from build123d import *

# Parameters (mm, degrees)
F0_W     = 19.05
F0_H     = 152.4
F0_W_2   = 304.8
F0_H_2   = 38.1
F1_DEPTH = 19.05


with BuildPart() as f1:
    # F0 (on Front) → F1 (new body)
    with BuildSketch(Plane.XZ):
        Polygon((-438.15, -314.325), (-438.15, -447.675), (-152.4, -447.675), (152.4, -447.675), (438.15, -447.675), (438.15, -314.325), (438.15, -161.925), (438.15, 142.875), (438.15, 295.275), (438.15, 447.675), (357.716667, 447.675), (357.716667, 422.275), (338.666667, 422.275), (338.666667, 447.675), (258.233333, 447.675), (258.233333, 422.275), (239.183333, 422.275), (239.183333, 447.675), (158.75, 447.675), (158.75, 422.275), (139.7, 422.275), (139.7, 447.675), (59.266667, 447.675), (59.266667, 422.275), (40.216667, 422.275), (40.216667, 447.675), (-40.216667, 447.675), (-40.216667, 422.275), (-59.266667, 422.275), (-59.266667, 447.675), (-139.7, 447.675), (-139.7, 422.275), (-158.75, 422.275), (-158.75, 447.675), (-239.183333, 447.675), (-239.183333, 422.275), (-258.233333, 422.275), (-258.233333, 447.675), (-338.666667, 447.675), (-338.666667, 422.275), (-357.716667, 422.275), (-357.716667, 447.675), (-438.15, 447.675), (-438.15, 295.275), (-438.15, 142.875), (-438.15, -161.925), align=None)
        Polygon((-304.00625, -193.675), (-304.00625, -117.475), (305.59375, -117.475), (305.59375, -193.675), (305.59375, -231.775), (286.54375, -231.775), (286.54375, -193.675), (207.16875, -193.675), (207.16875, -231.775), (188.11875, -231.775), (188.11875, -193.675), (108.74375, -193.675), (108.74375, -231.775), (89.69375, -231.775), (89.69375, -193.675), (10.31875, -193.675), (10.31875, -231.775), (-8.73125, -231.775), (-8.73125, -193.675), (-88.10625, -193.675), (-88.10625, -231.775), (-107.15625, -231.775), (-107.15625, -193.675), (-186.53125, -193.675), (-186.53125, -231.775), (-205.58125, -231.775), (-205.58125, -193.675), (-284.95625, -193.675), (-284.95625, -231.775), (-304.00625, -231.775), align=None, mode=Mode.SUBTRACT)
        with Locations((-447.675, 219.075)):
            Rectangle(F0_W, F0_H)
        with Locations((-447.675, -238.125)):
            Rectangle(F0_W, F0_H)
        with Locations((0, -466.725)):
            Rectangle(F0_W_2, F0_H_2)
        with Locations((447.675, -238.125)):
            Rectangle(F0_W, F0_H)
        with Locations((447.675, 219.075)):
            Rectangle(F0_W, F0_H)
    extrude(amount=F1_DEPTH)


solid = f1.part
Could you check a few things on this model? Use its own coordinates, in mm. Give positions to 0.01 mm unless a question says otherwise; leave off trailing zeros. Loops run counter-clockwise (first coordinate to the right, second up) from the corner with the lowest first, then second, coordinate; pieces in that order, holes last. Notation, with made-up numbers: (76.25, 75) -> (100.25, 75) arc R13 cw to (100.25, 99) -> close; hole circle Ø5 at (52, 3). An arc over 180 degrees is marked (long way). Return JSON: item names as keys, results as strings.
Item 1: I'm going to push flat-ended pins straight in: pin 1 (9.5 mm diameter, centred on y = -5.5, z = 429, fed in from -X); pin 2 (5 mm diameter, centred on x = 259, y = -8.5, fed in from -Z) (3 decimals); pin 3 (1.5 mm diameter, centred on y = -15.5, z = 131, fed in from +X). Where does each tip first touch, or does it pass through?
Geometry results:
{"pin 1": "stops at x = -438.15", "pin 2": "stops at z = -447.675", "pin 3": "stops at x = 438.15"}
Item 2: If we section it at A-A on z = -175: List the corners of the cut face in (x, y) for me.
Geometry results:
{"outline": "(-457.2, -19.05) -> (-304.01, -19.05) -> (-304.01, 0) -> (-457.2, 0) -> close; (305.59, -19.05) -> (457.2, -19.05) -> (457.2, 0) -> (305.59, 0) -> close"}
Item 3: I need wall thicknesses on L1, parallel to Z at x = 248, y = -1 (3 decimals); L2, parallel to Z at x = 160, y = -9.25 (3 decimals); L3, parallel to X at y = -4.75, z = -130.5. Which ranges of each line are inside material? Lowest first, please. Write a range as from..to.
Geometry results:
{"L1": "z = -447.675..-193.675, -117.475..422.275", "L2": "z = -447.675..-193.675, -117.475..447.675", "L3": "x = -438.15..-304.01, 305.59..438.15"}
Item 4: If we section it at B-B on x = -20.5: List the corners of the cut face in (y, z) for me (3 decimals).
Geometry results:
{"outline": "(-19.05, -485.775) -> (0, -485.775) -> (0, -193.675) -> (-19.05, -193.675) -> close; (-19.05, -117.475) -> (0, -117.475) -> (0, 447.675) -> (-19.05, 447.675) -> close"}
